from build123d import *

# Parameters (mm, degrees)
BOSS_EXTRU_1_DEPTH = 80


with BuildPart() as part:
    # Esquisse1 → Boss.-Extru.1 (new body)
    with BuildSketch(Plane.XY):
        with BuildLine():
            Line((2.9, 0), (0.1, 0))
            Line((0.1, 0), (0.1, -14))
            ThreePointArc((0.1, -14), (0.363603897, -14.636396103), (1, -14.9))
            Line((1, -14.9), (2.585786438, -14.9))
            ThreePointArc((2.585786438, -14.9), (2.930201527, -14.831491579), (3.222182541, -14.636396103))
            Line((3.222182541, -14.636396103), (9.586143571, -8.272435072))
            ThreePointArc((9.586143571, -8.272435072), (9.849747468, -7.636038969), (9.586143571, -6.999642866))
            Line((9.586143571, -6.999642866), (8.87903679, -6.292536085))
            ThreePointArc((8.87903679, -6.292536085), (8.242640687, -6.028932188), (7.606244584, -6.292536085))
            Line((7.606244584, -6.292536085), (4.777817459, -9.12096321))
            ThreePointArc((4.777817459, -9.12096321), (3.579048224, -9.359413236), (2.9, -8.343145751))
            Line((2.9, -8.343145751), (2.9, 0))
        make_face()
        with BuildLine():
            Line((0.1, 14), (0.1, 0))
            Line((0.1, 0), (2.9, 0))
            Line((2.9, 0), (2.9, 8.343145751))
            ThreePointArc((2.9, 8.343145751), (3.579048224, 9.359413236), (4.777817459, 9.12096321))
            Line((4.777817459, 9.12096321), (7.606244584, 6.292536085))
            ThreePointArc((7.606244584, 6.292536085), (8.242640687, 6.028932188), (8.87903679, 6.292536085))
            Line((8.87903679, 6.292536085), (9.586143571, 6.999642866))
            ThreePointArc((9.586143571, 6.999642866), (9.849747468, 7.636038969), (9.586143571, 8.272435072))
            Line((9.586143571, 8.272435072), (3.222182541, 14.636396103))
            ThreePointArc((3.222182541, 14.636396103), (2.930201527, 14.831491579), (2.585786438, 14.9))
            Line((2.585786438, 14.9), (1, 14.9))
            ThreePointArc((1, 14.9), (0.363603897, 14.636396103), (0.1, 14))
        make_face()
    extrude(amount=BOSS_EXTRU_1_DEPTH)


solid = part.part
Could you check a few things on this model? Use its own coordinates, in mm. A direction names the side the tool comes from. Round coordinates to 2 decimals unless told otherwise and drop trailing zeros. Order: outer loops, then holes, each group sorted by start corner. A loop starts at its lowest first (then second) coordinate and runs counter-clockwise, first axis right, second up.
(1) If we mould it in two halves opening along Y, with no side actions, what happens to faces 1 (the flat face through (2.7, 0.2, 80)), 2 (the flat face through (6.36, -11.5, 39.44)), 3 (the flat face through (6.45, 11.41, 39.44)), 4 (the flat face through (6.2, -7.7, 39.4))? For each: released by +Y, released by -Y, zero draft, split by the parting line, or undercut.
Response values:
face 1: zero draft
face 2: released by -Y
face 3: released by +Y
face 4: undercut
(2) I'm going to push flat-ended pins straight in: pin 1 (1.5 mm diameter, centred on x = 3.5, z = 29, fed in from +Y); pin 2 (12 mm diameter, centred on y = -0.5, z = 34.5, fed in from +X); pin 3 (2 mm diameter, centred on x = 5.5, z = 41, fed in from -Y). Where does each tip first touch, or does it pass through?
Response values:
pin 1: stops at y = 14.88
pin 2: stops at x = 9.09
pin 3: stops at y = -13.36
(3) Which directions (+Z, -Z, +X, -X, +Y, -Y) give clear straight access to the entire face, cutting with the end or side of a thin tool? Please do faces 5 (the flat face through (2.9, 0, 39)), 6 (the flat face through (2.7, 0.2, 0)).
Response values:
face 5: +Z, -Z
face 6: -Z, +X, -X, +Y, -Y
(4) Imagine slicing it at D-D (y = 12.5). Write out the boundary of the cut face in (x, z), plus the area to 3 significant figures.
Response values:
outline: (0.1, 0) - (5.36, 0) - (5.36, 80) - (0.1, 80) - close
area: 421 mm2
(5) Imagine slicing it at B-B (z = 33). Write out the boundary of the cut face in (x, y).
Response values:
outline: (0.1, -14) arc R0.9 ccw to (1, -14.9) - (2.59, -14.9) arc R0.9 ccw to (3.22, -14.64) - (9.59, -8.27) arc R0.9 ccw to (9.59, -7) - (8.88, -6.29) arc R0.9 ccw to (7.61, -6.29) - (4.78, -9.12) arc R1.1 cw to (2.9, -8.34) - (2.9, 8.34) arc R1.1 cw to (4.78, 9.12) - (7.61, 6.29) arc R0.9 ccw to (8.88, 6.29) - (9.59, 7) arc R0.9 ccw to (9.59, 8.27) - (3.22, 14.64) arc R0.9 ccw to (2.59, 14.9) - (1, 14.9) arc R0.9 ccw to (0.1, 14) - close
(6) Please list where these lines run through material, in increasing order: line 1 along Y through (x, z) = (3.75, 71); line 2 along X through (y, z) = (-7.75, 17); line 3 along Y through (x, z) = (4.5, 60).
Response values:
line 1: y = -14.11 to -9.41, 9.41 to 14.11
line 2: x = 0.1 to 2.9, 6.15 to 9.84
line 3: y = -13.36 to -9.32, 9.32 to 13.36
(7) Imagine slicing it at A-A (x = 6.5). Write out the boundary of the cut face in (y, z).
Response values:
outline: (-11.36, 0) - (-7.4, 0) - (-7.4, 80) - (-11.36, 80) - close; (7.4, 0) - (11.36, 0) - (11.36, 80) - (7.4, 80) - close
(8) Imagine slicing it at C-C (y = -5.25). Write out the boundary of the cut face in (x, z), plus the area to 3 significant figures.
Response values:
outline: (0.1, 0) - (2.9, 0) - (2.9, 80) - (0.1, 80) - close
area: 224 mm2
